```python
from build123d import *

# Parameters (mm, degrees)
SKETCH_1_W          = 2540
SKETCH_1_H          = 100
EXTRUDE_453_DEPTH   = 12
SKETCH_2_W          = 2540
SKETCH_2_H          = 12
EXTRUDE_1_DEPTH     = 86
CUT_EXTRUDE_1_DEPTH = 1278.694799238


with BuildPart() as part:
    # 草图1 → Extrude 453 (new body)
    with BuildSketch(Plane.XY):
        Rectangle(SKETCH_1_W, SKETCH_1_H)
    extrude(amount=EXTRUDE_453_DEPTH)

    # 草图2 → 凸台-拉伸1 (add)
    with BuildSketch(Plane.XY.offset(12)):
        with Locations((0, 44)):
            Rectangle(SKETCH_2_W, SKETCH_2_H)
    extrude(amount=EXTRUDE_1_DEPTH)

    # 草图4 → 切除-拉伸1 (cut, through all)
    with BuildSketch(Plane(origin=(0, 50, 0), x_dir=(-1, 0, 0), z_dir=(0, 1, 0))):
        Polygon((-1270, 0), (-1270, 98), (-1000, 98), align=None)
        Polygon((1270, 0), (1000, 98), (1270, 98), align=None)
    extrude(amount=-CUT_EXTRUDE_1_DEPTH, mode=Mode.SUBTRACT)


solid = part.part
```
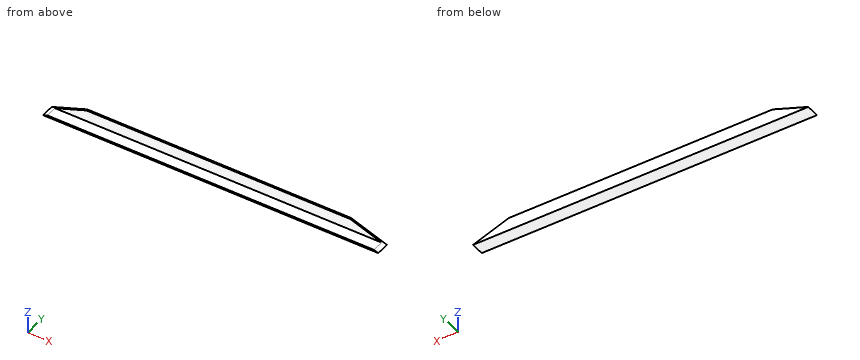
Here's how the part is built. I have some questions about the finished solid (model axes, mm). Coordinates: 2 decimals unless noted, no trailing zeros. Loops run counter-clockwise (first coordinate to the right, second up) from the corner with the lowest first, then second, coordinate; pieces in that order, holes last. Notation, with made-up numbers: M -24.75,59.25 L 16.25,59.25 A11 cw 16.25,69.25 Z; hole C -5,84.25 d8. An arc over 180 degrees is marked long. One line per item, written item: value.
1. Please list where these lines run through material, in increasing order: probe 1 along Y at (x, z) = (948, 41.5); probe 2 along Z at (x, y) = (310, 14); probe 3 along Z at (x, y) = (1096.5, 42).
Geometry says:
probe 1: y = 38 to 50
probe 2: z = 0 to 12
probe 3: z = 0 to 62.97
2. Will these pins go through, and if not, where does the flat tip stop? pin 1 Ø8 at (x, z) = (306.5, 64) entering from -Y; pin 2 Ø10 at (x, y) = (-51, 10.5) entering from +Z.
Geometry says:
pin 1: stops at y = 38
pin 2: stops at z = 12
3. Imagine slicing it at C-C (z = 54). List the corners of the cut face in (x, y) for me, and give its area (3 significant figures).
Geometry says:
outline: M -1121.22,38 L 1121.22,38 L 1121.22,50 L -1121.22,50 Z
area: 26,900 mm2
4. Imagine slicing it at B-B (y = -9). List the corners of the cut face in (x, z) for me.
Geometry says:
outline: M -1270,0 L 1270,0 L 1236.94,12 L -1236.94,12 Z
5. Imagine slicing it at A-A (x = 745). List the corners of the cut face in (y, z) for me, and give its area (3 significant figures).
Geometry says:
outline: M -50,0 L 50,0 L 50,98 L 38,98 L 38,12 L -50,12 Z
area: 2,230 mm2
